Can you work these out from the model? Positions are in its coordinate system, mm. Round coordinates to 2 decimals unless told otherwise and drop trailing zeros. Write each loop counter-clockwise with the first axis right and the second up, starting at its lowest first coordinate (ties: lowest second). Pieces come first, ordered by that corner, then holes. Notation, with made-up numbers: M -16.75,44 L 37.25,44 A22 cw 37.25,79 Z; hole C -34.5,83.5 d3. An arc over 180 degrees is marked long. Answer in a Markdown table with one row per item. Add a question column.
(1) Suppose I cut it at A-A, the plane x = 50. Write out the boundary of the cut face in (y, z).
(2) Suppose I cut it at B-B, the plane y = 10. Write out the boundary of the cut face in (x, z).
(3) Suppose I cut it at C-C, the plane z = 3.85. Count the separate pieces of the cut face and the enclosed holes in it, then the cut area to 3 significant figures.
(4) I'm going to push flat-ended pins straight in: pin 1 (1.5 mm diameter, centred on y = -80.5, z = 3, fed in from -X); pin 2 (3 mm diameter, centred on x = 101, z = 4.5, fed in from -Y). Where does each tip first touch, or does it pass through?
(5) Suppose I cut it at D-D, the plane x = 30. Write out the boundary of the cut face in (y, z).
(6) If I drill on probe 1 along X at (y, z) = (-5.5, 3.05); probe 2 along X at (y, z) = (-65, 2.95); probe 3 along Y at (x, z) = (95, 3.15), over which ranges is the centre line in solid material (lowest first)?
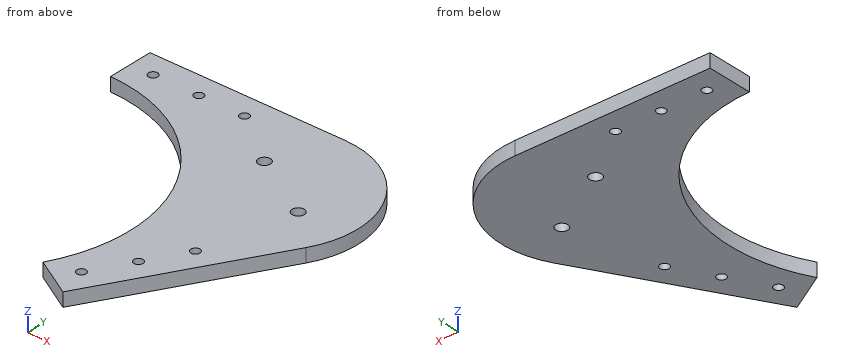
from build123d import *

# Parameters (mm, degrees)
EXTRUDE_1_DEPTH          = 6
FILLET_1_R               = 70
FILLET_2_R               = 40
CUT_EXTRUDE_1_DEPTH      = 170.497303225
CUT_EXTRUDE_1_DEPTH_BACK = 170.497303225
SKETCH_2_R               = 2.65
SKETCH_3_R               = 2
CUT_EXTRUDE_2_DEPTH      = 10


with BuildPart() as part:
    # 草图1 → 凸台-拉伸1 (new body)
    with BuildSketch(Plane.XY):
        Polygon((0, 0), (120, 0), (60, -103.923048454), (77.320508076, -113.923048454), (154.641016151, 20), (0, 20), align=None)
    extrude(amount=EXTRUDE_1_DEPTH)

    # 圆角1
    # the kernel refuses this fillet: 70 mm, written as the material it adds along each edge
    with BuildSketch(Plane(origin=(120, 0, 0), x_dir=(-1, 0, 0), z_dir=(0, 0, 1))) as fillet_1_piece_1:
        with BuildLine():
            CenterArc((121.224989992, 69.989280604), FILLET_1_R, 151.002719134, 117.994561732)
            Line((60, 103.923048454), (0, 0))
            Line((0, 0), (120, 0))
        make_face()
    extrude(amount=6)

    # 圆角2
    fillet_2_edges = [part.edges().sort_by_distance(p)[0] for p in [
        (154.641016151, 20, 3),
    ]]
    fillet(fillet_2_edges, radius=FILLET_2_R)

    # 草图2 → 切除-拉伸1 (cut, two sides: drawn at the far end of the back side and taken through both)
    with BuildSketch(Plane.XY.offset(6).offset(-CUT_EXTRUDE_1_DEPTH_BACK)):
        with Locations((103.232600298, -24.545834576)):
            Circle(SKETCH_2_R)
        with Locations((73.787736569, -7.545834576)):
            Circle(SKETCH_2_R)
    extrude(amount=CUT_EXTRUDE_1_DEPTH + CUT_EXTRUDE_1_DEPTH_BACK, mode=Mode.SUBTRACT)

    # 草图3 → 切除-拉伸2 (cut)
    with BuildSketch(Plane.XY.offset(6)):
        with Locations((10, 10)):
            Circle(SKETCH_3_R)
        with Locations((30, 10)):
            Circle(SKETCH_3_R)
        with Locations((50, 10)):
            Circle(SKETCH_3_R)
        with Locations((73.660254038, -100.262794416)):
            Circle(SKETCH_3_R)
        with Locations((83.660254038, -82.942286341)):
            Circle(SKETCH_3_R)
        with Locations((93.660254038, -65.621778265)):
            Circle(SKETCH_3_R)
    extrude(amount=-CUT_EXTRUDE_2_DEPTH, mode=Mode.SUBTRACT)


solid = part.part
Calculated:
| question | item | result |
|---|---|---|
| 1 | outline | M -22.28,0 L 8,0 L 8,6 L -22.28,6 Z; M 12,0 L 20,0 L 20,6 L 12,6 Z |
| 2 | outline | M 0,0 L 8,0 L 8,6 L 0,6 Z; M 12,0 L 28,0 L 28,6 L 12,6 Z; M 32,0 L 48,0 L 48,6 L 32,6 Z; M 52,0 L 111.82,0 L 111.82,6 L 52,6 Z |
| 3 | separate pieces | 1 |
| 3 | enclosed holes | 8 |
| 3 | area | 7,630 mm² |
| 4 | pin 1 | x = 67.86 |
| 4 | pin 2 | y = -75.51 |
| 5 | outline | M -7.34,0 L 8,0 L 8,6 L -7.34,6 Z; M 12,0 L 20,0 L 20,6 L 12,6 Z |
| 6 | probe 1 | 26 to 72.1, 75.47 to 122.64 |
| 6 | probe 2 | 68.6 to 91.76, 95.56 to 105.57 |
| 6 | probe 3 | -83.3 to -67.11, -64.14 to 18.82 |
